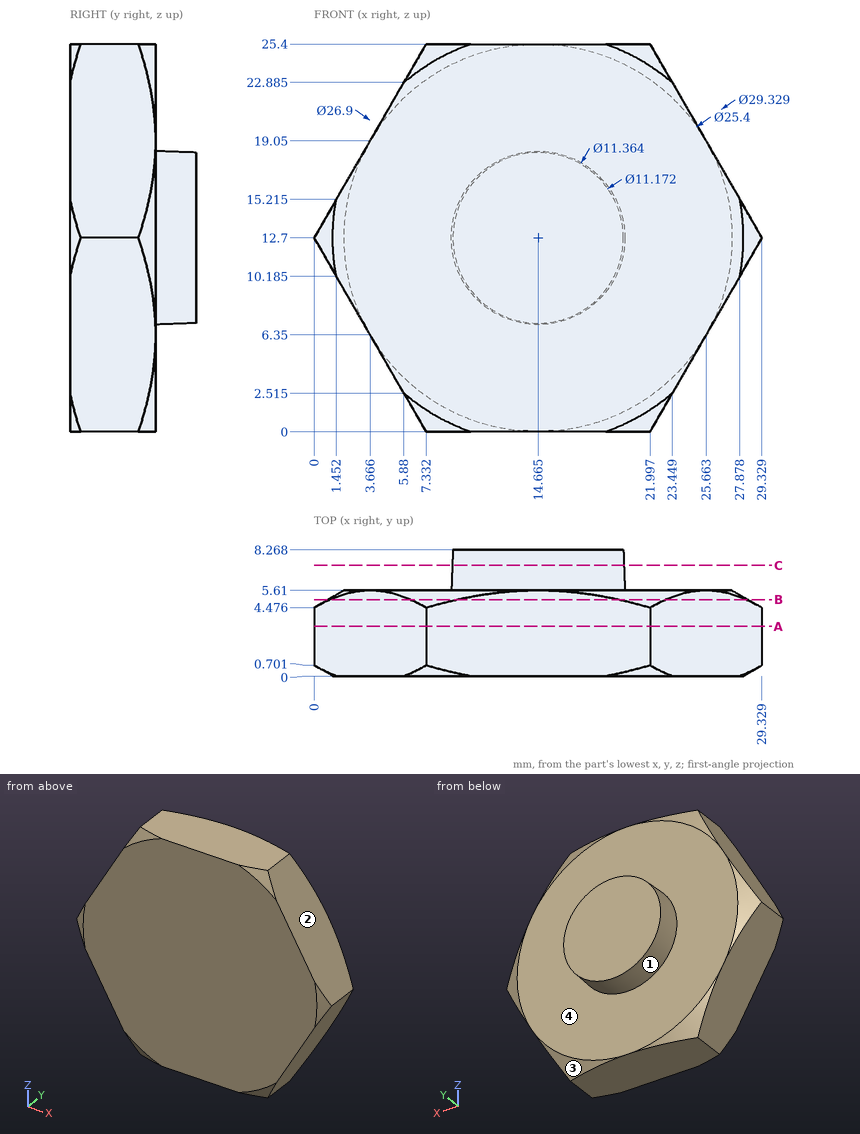
Geometry: see drawing. Coordinates: mm, zero at the bounding-box minimum. Give positions to 0.01 mm unless a question says otherwise; leave off trailing zeros. Write each loop counter-clockwise with the first axis right and the second up, starting at its lowest first coordinate (ties: lowest second). Pieces come first, ordered by that corner, then holes. Notation, with made-up numbers: M -26,80 L -8,80 A25 ccw -8,93 Z; hole C -29,64.5 d11. An arc over 180 degrees is marked long. Answer as a JSON object with one key per item and string values.
Q1. Cut plane B-B, the plane y = 5. Return the cut outline in (x, z) (1 decimal).
Geometry check:
{"outline": "M 1,10.9 L 6.3,1.8 A13.8 ccw 9.4,0 L 20,0 A13.8 ccw 23,1.8 L 28.3,10.9 A13.8 ccw 28.3,14.5 L 23,23.6 A13.8 ccw 20,25.4 L 9.4,25.4 A13.8 ccw 6.3,23.6 L 1,14.5 A13.8 ccw Z"}
Q2. Cut plane A-A, the plane y = 3.25. Return the cut outline in (x, z).
Geometry check:
{"outline": "M 0,12.7 L 7.33,0 L 22,0 L 29.33,12.7 L 22,25.4 L 7.33,25.4 Z"}
Q3. Mould query, pull axis Z, two halves, no side actions, for the marked faces 1, 2, 3 and 4. Classes: +Z half, -Z half, draft (parallel to the pull), parting line (faces both ways), or undercut.
Geometry check:
{"face 1": "parting line", "face 2": "+Z half", "face 3": "-Z half", "face 4": "draft"}
Q4. Ray query, line 1 along Y through (x, z) = (9.5, 5.75); line 2 along Z through (x, y) = (3.5, 4.25) (1 decimal); line 3 along X through (y, z) = (1.75, 1.5) (1 decimal). Return the intervals inside material, ascending.
Geometry check:
{"line 1": "y = 0 to 5.61", "line 2": "z = 6.6 to 18.8", "line 3": "x = 6.5 to 22.9"}
Q5. Cut plane C-C, the plane y = 7.25. Return the cut outline in (x, z) (1 decimal).
Geometry check:
{"outline": "C 14.7,12.7 d11.2"}
